Source: three-view drawing plus pictorial views. Frame: mm from the lowest corner of the part. Give positions to 0.01 mm unless a question says otherwise; leave off trailing zeros. Loops run counter-clockwise (first coordinate to the right, second up) from the corner with the lowest first, then second, coordinate; pieces in that order, holes last. Notation, with made-up numbers: (-5.75, 0.5) - (19.25, 0.5) arc R4 ccw to (19.25, 6.5) - close; hole circle Ø1 at (42.25, -24). An arc over 180 degrees is marked (long way). Write each question's results on one line, items separated by ' | '. Start each with the question number.
(1) Cut plane A-A on y = 1.8. Return the cut outline in (x, z), then the cut area to 3 significant figures.
(2) Contact query for flat-ended pins moving along their axis: pin 1 (2.5 mm diameter, centred on x = 72.5, y = 2.5, fed in from -Z); pin 2 (2.5 mm diameter, centred on y = 1.5, z = 2, fed in from +X); pin 3 (1 mm diameter, centred on x = 74.5, y = 4, fed in from +Z); pin 4 (0.9 mm diameter, centred on y = 1.5, z = 2, fed in from -X). Output: stop coordinate, or through.
(3) Material intervals for line 1 along X through (y, z) = (2.7, 15.75); line 2 along Z through (x, y) = (30, 1.5); line 3 along Z through (x, y) = (163, 2), sorted ascending. Write a range as [from, to].
(4) Cut plane B-B on x = 154. Return the cut outline in (y, z).
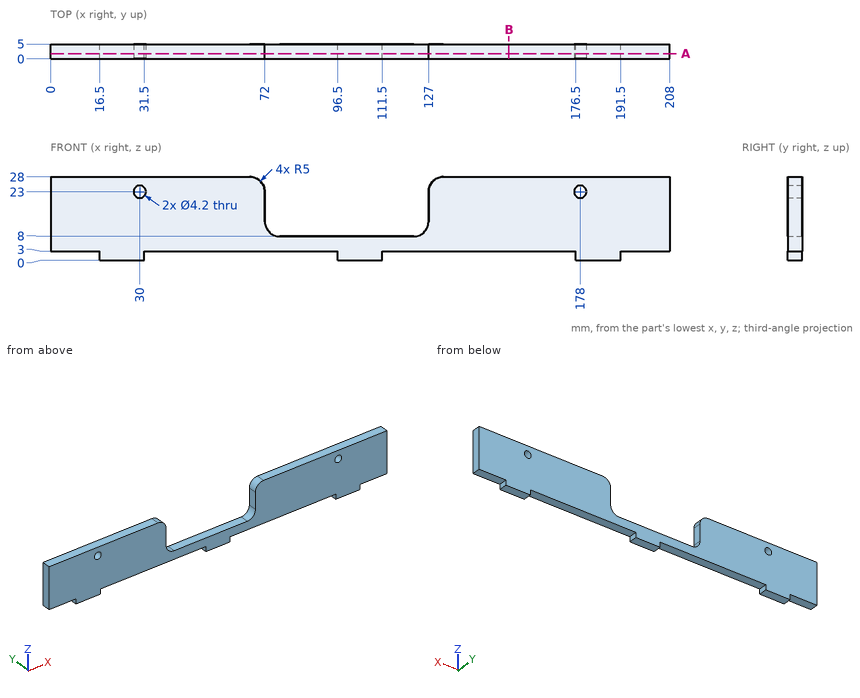
Ans:
1) outline: (0, 3) - (16.5, 3) - (16.5, 0) - (31.5, 0) - (31.5, 3) - (96.5, 3) - (96.5, 0) - (111.5, 0) - (111.5, 3) - (176.5, 3) - (176.5, 0) - (191.5, 0) - (191.5, 3) - (208, 3) - (208, 28) - (132, 28) arc R5 ccw to (127, 23) - (127, 13) arc R5 cw to (122, 8) - (77, 8) arc R5 cw to (72, 13) - (72, 23) arc R5 ccw to (67, 28) - (0, 28) - close; hole circle Ø4.2 at (30, 23); hole circle Ø4.2 at (178, 23) | area: 4,210 mm^2
2) pin 1: z = 3 | pin 2: x = 208 | pin 3: z = 9 | pin 4: x = 16.5
3) line 1: [0, 72], [127, 208] | line 2: [0, 20.9], [25.1, 28] | line 3: [3, 28]
4) outline: (0, 3) - (5, 3) - (5, 28) - (0, 28) - close
